from build123d import *

# Parameters (mm, degrees)
SKETCH1_W           = 14.224
SKETCH1_H           = 3.175
SKETCH1_W_2         = 19.05
SKETCH1_R           = 1.5875
SKETCH1_W_3         = 13.6398
SKETCH1_H_2         = 9.144
BOSS_EXTRUDE1_DEPTH = 3.175
SKETCH2_R           = 1.5875
CUT_EXTRUDE1_DEPTH  = 3.175
CUT_EXTRUDE2_DEPTH  = 251.18113563


with BuildPart() as part:
    # Sketch1 → Boss-Extrude1 (new body)
    with BuildSketch(Plane(origin=(0, 0, 0), x_dir=(1, 0, 0), z_dir=(0, 1, 0))):
        Polygon((0, 101.6), (0, 0), (50.8, 0), (50.8, 3.175), (65.024, 3.175), (65.024, 0), (228.6, 0), (228.6, 101.6), (65.024, 101.6), (65.024, 98.425), (50.8, 98.425), (50.8, 101.6), align=None)
        with Locations((57.912, 23.6855)):
            Rectangle(SKETCH1_W, SKETCH1_H, mode=Mode.SUBTRACT)
        with Locations((32.512, 33.2105)):
            Rectangle(SKETCH1_W_2, SKETCH1_H, mode=Mode.SUBTRACT)
        with Locations((83.312, 33.2105)):
            Rectangle(SKETCH1_W_2, SKETCH1_H, mode=Mode.SUBTRACT)
        with Locations(Location((99.187, 30.48, 0), (0, 0, 270))):
            Circle(SKETCH1_R, mode=Mode.SUBTRACT)
        with Locations(Location((147.701, 30.48, 0), (0, 0, 270))):
            Circle(SKETCH1_R, mode=Mode.SUBTRACT)
        with Locations(Location((162.814, 39.6875, 0), (0, 0, 270))):
            Circle(SKETCH1_R, mode=Mode.SUBTRACT)
        with Locations(Location((190.91275, 39.6875, 0), (0, 0, 270))):
            Circle(SKETCH1_R, mode=Mode.SUBTRACT)
        with Locations((32.512, 68.3895)):
            Rectangle(SKETCH1_W_2, SKETCH1_H, mode=Mode.SUBTRACT)
        with Locations((83.312, 68.3895)):
            Rectangle(SKETCH1_W_2, SKETCH1_H, mode=Mode.SUBTRACT)
        with Locations((57.912, 77.9145)):
            Rectangle(SKETCH1_W, SKETCH1_H, mode=Mode.SUBTRACT)
        with Locations(Location((104.14, 82.931, 0), (0, 0, 270))):
            Circle(SKETCH1_R, mode=Mode.SUBTRACT)
        with Locations(Location((162.814, 61.9125, 0), (0, 0, 270))):
            Circle(SKETCH1_R, mode=Mode.SUBTRACT)
        with Locations(Location((190.91275, 61.9125, 0), (0, 0, 270))):
            Circle(SKETCH1_R, mode=Mode.SUBTRACT)
        with Locations(Location((139.319, 82.931, 0), (0, 0, 270))):
            Circle(SKETCH1_R, mode=Mode.SUBTRACT)
        with Locations((123.444, 93.853)):
            Rectangle(SKETCH1_W_3, SKETCH1_H_2, mode=Mode.SUBTRACT)
    extrude(amount=BOSS_EXTRUDE1_DEPTH)

    # Sketch2 → Cut-Extrude1 (cut)
    with BuildSketch(Plane(origin=(0, 3.175, 0), x_dir=(1, 0, 0), z_dir=(0, 1, 0))):
        with Locations(Location((15.24, 60.325, 0), (0, 0, 270))):
            Circle(SKETCH2_R)
        with Locations(Location((15.24, 41.275, 0), (0, 0, 270))):
            Circle(SKETCH2_R)
        with Locations(Location((21.59, 41.275, 0), (0, 0, 270))):
            Circle(SKETCH2_R)
        with Locations(Location((21.59, 60.325, 0), (0, 0, 270))):
            Circle(SKETCH2_R)
    extrude(amount=-CUT_EXTRUDE1_DEPTH, mode=Mode.SUBTRACT)

    # Sketch3 → Cut-Extrude2 (cut, through all)
    with BuildSketch(Plane(origin=(0, 3.175, 0), x_dir=(1, 0, 0), z_dir=(0, 1, 0))):
        Polygon((0, 63.5), (31.75, 101.6), (0, 101.6), align=None)
        Polygon((152.4, 101.6), (205.74, 69.85), (205.74, 31.75), (152.4, 0), (228.6, 0), (228.6, 44.45), (228.6, 57.15), (228.6, 101.6), align=None)
        Polygon((31.75, 0), (0, 0), (0, 38.1), align=None)
    extrude(amount=-CUT_EXTRUDE2_DEPTH, mode=Mode.SUBTRACT)


solid = part.part
Can you work these out from the model? Positions are in its coordinate system, mm. Coordinates: 2 decimals unless noted, no trailing zeros. Loops run counter-clockwise (first coordinate to the right, second up) from the corner with the lowest first, then second, coordinate; pieces in that order, holes last. Notation, with made-up numbers: M 84.25,-3 L 137.25,-3 A30 cw 137.25,31 Z; hole C 46,57.5 d3. An arc over 180 degrees is marked long. Answer as CSV lines item,"result". Start each with the question number.
1. Suppose I cut it at A-A, the plane x = 29. List the corners of the cut face in (y, z) for me (3 decimals).
2. Suppose I cut it at C-C, the plane y = 1. Count the separate pieces of the cut face and the enclosed holes in it, plus the area to 3 significant figures.
3. Suppose I cut it at B-B, the plane z = -19. List the corners of the cut face in (x, y) for me (3 decimals), plus the area to 3 significant figures.
4. For pin 1 Ø1 at (y, z) = (2, -68.5) entering from -X; pin 2 Ø1 at (y, z) = (2.5, -21.5) entering from +X, each with a flat end and sliding along its axis, tell me the tip position at first contact or that it passes through.
5. If I drill on probe 1 along Z at (x, y) = (90.5, 0.85); probe 2 along Z at (x, y) = (23.5, 0.2); probe 3 along X at (y, z) = (2.85, -69.5), over which ranges is the centre line in solid material (lowest first)? Write a range as [from, to].
Output:
1,outline,"M 0,-98.3 L 3.175,-98.3 L 3.175,-69.977 L 0,-69.977 Z; M 0,-66.802 L 3.175,-66.802 L 3.175,-34.798 L 0,-34.798 Z; M 0,-31.623 L 3.175,-31.623 L 3.175,-3.3 L 0,-3.3 Z"
2,separate pieces,"1"
2,enclosed holes,"19"
2,area,"17,400 mm^2"
3,outline,"M 15.917,0 L 184.32,0 L 184.32,3.175 L 15.917,3.175 Z"
3,area,"535 mm^2"
4,pin 1,"stops at x = 3.75"
4,pin 2,"stops at x = 189.36"
5,probe 1,"z = [-101.6, -69.98], [-66.8, -34.8], [-31.62, 0]"
5,probe 2,"z = [-91.7, -69.98], [-66.8, -34.8], [-31.62, -9.9]"
5,probe 3,"x = [5, 22.99], [42.04, 73.79], [92.84, 205.74]"
